from build123d import *

# Parameters (mm, degrees)
SKETCH1_W           = 6.985
SKETCH1_H           = 1.905
BOSS_EXTRUDE1_DEPTH = 12.7
FILLET1_R           = 1.27


with BuildPart() as part:
    # Sketch1 → Boss-Extrude1 (new body)
    with BuildSketch(Plane.XY):
        with BuildLine():
            add(Edge.make_bspline(
                [(5.3975, 4.482325921), (0, 8.995887562), (-5.3975, 4.482325921)],
                knots=[3.925254702, 3.925254702, 3.925254702, 5.499523258, 5.499523258, 5.499523258], degree=2, weights=[1, 0.705878098, 1]))
            Line((5.3975, 4.482325921), (5.3975, 12.065))
            Line((5.3975, 12.065), (-5.3975, 12.065))
            Line((-5.3975, 12.065), (-5.3975, 4.482325921))
        make_face()
        with Locations((0, 9.2075)):
            Rectangle(SKETCH1_W, SKETCH1_H, mode=Mode.SUBTRACT)
    extrude(amount=BOSS_EXTRUDE1_DEPTH)

    # Fillet1
    fillet1_edges = [part.edges().sort_by_distance(p)[0] for p in [
        (-5.3975, 12.065, 6.35),
        (5.3975, 12.065, 6.35),
    ]]
    fillet(fillet1_edges, radius=FILLET1_R)


solid = part.part
For this review, take the finished solid that the model builds, in its own axes (mm). A direction names the side the tool comes from. Coordinates: 2 decimals unless noted, no trailing zeros. Order: outer loops, then holes, each group sorted by start corner. A loop starts at its lowest first (then second) coordinate and runs counter-clockwise, first axis right, second up. Notation, with made-up numbers: (25, 73) - (53, 73) arc R31 ccw to (53, 97) - close; hole circle Ø4 at (73.25, -15.75). An arc over 180 degrees is marked (long way). Answer as CSV lines item,"result". Start each with the question number.
1) Machinability: for faces 5 (the flat face through (0, 12.065, 6)), 6 (the flat face through (0, 8.255, 6)), which of the approach directions +Z, -Z, +X, -X, +Y, -Y give a long, thin tool a straight path to every point of the face, cutting with its end or side? Answer none if there is none.
2) To check wall thickness, follow line 1 along X through (y, z) = (9.5, 11.5); line 2 along Y through (x, z) = (0, 8) (3 decimals); line 3 along X through (y, z) = (5, 8.75). State the ranges of each line that lie inside material, in increasing order. Write a range as [from, to].
3) Draft analysis for pull direction X (two halves, no side actions). For faces 1 (the flat face through (-3.492, 9, 6)), 2 (the flat face through (0, 10.16, 6)), 3 (the flat face through (-5.398, 8, 6)), 4 (the flat face through (0, 7, 12.7)), state which applies: +X half, -X half, draft (parallel to the pull), parting line (faces both ways), or undercut.
4) Add section A-A (y = 8.75). State the section outline as (x, z) points, then the cut area to 3 significant figures.
5) Insertion check: P1, Ø3.5, axis at x = -1, z = 4.5, coming from the -Y side. The pin has a flat end and moves straight along its axis. Give the tip position at first contact, or say it passes through.
Result:
1,face 5,"+Z, -Z, +X, -X, +Y"
1,face 6,"+Z, -Z"
2,line 1,"[-5.4, -3.49], [3.49, 5.4]"
2,line 2,"[6.35, 8.255], [10.16, 12.065]"
2,line 3,"[-5.4, -4.7], [4.7, 5.4]"
3,face 1,"undercut"
3,face 2,"undercut"
3,face 3,"-X half"
3,face 4,"draft"
4,outline,"(-5.4, 0) - (-3.49, 0) - (-3.49, 12.7) - (-5.4, 12.7) - close; (3.49, 0) - (5.4, 0) - (5.4, 12.7) - (3.49, 12.7) - close"
4,area,"48.4 mm^2"
5,P1,"y = 5.92"
